```python
from build123d import *

# Parameters (mm, degrees)
ARMB_W_DEPTH             = 19.5
FILLET_1_R               = 16
FILLET_2_R               = 10
CUT_EXTRUDE_1_DEPTH      = 169.89419765
CUT_EXTRUDE_1_DEPTH_BACK = 169.89419765
SKETCH_2_R               = 10
CUT_EXTRUDE_2_DEPTH      = 169.89419765
CUT_EXTRUDE_2_DEPTH_BACK = 169.89419765
ARMB_T_W                 = 35
ARMB_T_H                 = 18
CUT_EXTRUDE_3_DEPTH      = 169.89419765
SKETCH_5_R               = 4
SKETCH_5_R_2             = 3.25
CUT_EXTRUDE_4_DEPTH      = 173.238207143
SKETCH_6_R               = 3
CUT_EXTRUDE_5_DEPTH      = 171.133036181
CHAMFER_1_SIZE           = 0.2


with BuildPart() as part:
    # ArmB-L → ArmB-W (new, symmetric)
    with BuildSketch(Plane.XY):
        with BuildLine():
            Line((12.489995997, 10), (167, 10))
            Line((167, 10), (167, -10))
            Line((167, -10), (12.489995997, -10))
            ThreePointArc((12.489995997, -10), (-16, 0), (12.489995997, 10))
        make_face()
    extrude(amount=ARMB_W_DEPTH, both=True)

    # ﾌｨﾚｯﾄ1
    fillet_1_edges = [part.edges().sort_by_distance(p)[0] for p in [
        (167, 10, 0),
    ]]
    fillet(fillet_1_edges, radius=FILLET_1_R)

    # ﾌｨﾚｯﾄ2
    fillet_2_edges = [part.edges().sort_by_distance(p)[0] for p in [
        (12.489995997, 10, 0),
        (12.489995997, -10, 0),
    ]]
    fillet(fillet_2_edges, radius=FILLET_2_R)

    # ｽｹｯﾁ2 → ｶｯﾄ - 押し出し1 (cut, two sides: drawn at the far end of the back side and taken through both)
    with BuildSketch(Plane.XY.offset(-CUT_EXTRUDE_1_DEPTH_BACK)):
        Circle(SKETCH_2_R)
    extrude(amount=CUT_EXTRUDE_1_DEPTH + CUT_EXTRUDE_1_DEPTH_BACK, mode=Mode.SUBTRACT)

    # ｽｹｯﾁ3 → ｶｯﾄ - 押し出し2 (cut, two sides: drawn at the far end of the back side and taken through both)
    with BuildSketch(Plane(origin=(0, 0, 0), x_dir=(1, 0, 0), z_dir=(0, 1, 0)).offset(-CUT_EXTRUDE_2_DEPTH_BACK)):
        with BuildLine():
            Line((-16, 17.5), (18.424067706, 17.5))
            ThreePointArc((18.424067706, 17.5), (26, 0), (18.424067706, -17.5))
            Line((18.424067706, -17.5), (-16, -17.5))
            Line((-16, -17.5), (-16, 17.5))
        make_face()
    extrude(amount=CUT_EXTRUDE_2_DEPTH + CUT_EXTRUDE_2_DEPTH_BACK, mode=Mode.SUBTRACT)

    # ArmB-t → ｶｯﾄ - 押し出し3 (cut, through all)
    with BuildSketch(Plane(origin=(0, 0, 0), x_dir=(0, 0, -1), z_dir=(1, 0, 0))):
        with Locations((0, 1)):
            Rectangle(ARMB_T_W, ARMB_T_H)
    extrude(amount=CUT_EXTRUDE_3_DEPTH, mode=Mode.SUBTRACT)

    # ｽｹｯﾁ5 → ｶｯﾄ - 押し出し4 (cut, through all)
    with BuildSketch(Plane.XY.offset(19.5)):
        with Locations((155, 3)):
            Circle(SKETCH_5_R)
        with Locations((139, 5)):
            Circle(SKETCH_5_R_2)
    extrude(amount=-CUT_EXTRUDE_4_DEPTH, mode=Mode.SUBTRACT)

    # ｽｹｯﾁ6 → ｶｯﾄ - 押し出し5 (cut, through all)
    with BuildSketch(Plane.XZ.offset(10)):
        with Locations(Location((155, 0, 0), (0, 0, 270))):
            Circle(SKETCH_6_R)
        with Locations(Location((40, 0, 0), (0, 0, 270))):
            Circle(SKETCH_6_R)
    extrude(amount=-CUT_EXTRUDE_5_DEPTH, mode=Mode.SUBTRACT)

    # 面取り1
    chamfer_1_edges = [part.edges().sort_by_distance(p)[0] for p in [
        (167, -8, 19.5),
        (151, 3, -19.5),
        (151, 3, -17.5),
        (151, 3, 17.5),
        (151, 3, 19.5),
        (135.75, 5, -19.5),
        (135.75, 5, -17.5),
        (135.75, 5, 17.5),
        (135.75, 5, 19.5),
        (155, -8, 3),
        (155, -10, 3),
        (40, -8, 3),
        (40, -10, 3),
        (83.806623863, 10, -19.5),
        (83.806623863, 10, 19.5),
        (162.313708499, 5.313708499, -19.5),
        (162.313708499, 5.313708499, 19.5),
        (91.806623863, -10, -19.5),
        (91.806623863, -10, 19.5),
        (-16, 0, -19.5),
        (-16, 0, 19.5),
        (13.216416623, -10.594600569, -19.5),
        (13.216416623, -10.594600569, 19.5),
        (13.216416623, 10.594600569, -19.5),
        (13.216416623, 10.594600569, 19.5),
        (-10, 0, -19.5),
        (-10, 0, 19.5),
        (167, -8, -19.5),
        (26, -10, 0),
        (-10, 0, -17.5),
        (17.518657716, -10, -17.5),
        (13.216416623, -10.594600569, -17.5),
        (-16, 0, -17.5),
        (13.216416623, 10.594600569, -17.5),
        (83.806623863, 10, -17.5),
        (-10, 0, 17.5),
        (13.216416623, -10.594600569, 17.5),
        (17.518657716, -10, 17.5),
        (83.806623863, 10, 17.5),
        (13.216416623, 10.594600569, 17.5),
        (-16, 0, 17.5),
        (167, -10, 0),
        (162.313708499, 5.313708499, 17.5),
        (162.313708499, 5.313708499, -17.5),
        (26, -8, 0),
        (167, -7, -17.5),
        (167, -7, 17.5),
        (167, -8, 0),
    ]]
    chamfer(chamfer_1_edges, length=CHAMFER_1_SIZE)


solid = part.part
```
Work out the finished part from the listing and answer in its coordinate system (mm). A direction names the side the tool comes from. Give positions to 0.01 mm unless a question says otherwise; leave off trailing zeros. Loops run counter-clockwise (first coordinate to the right, second up) from the corner with the lowest first, then second, coordinate; pieces in that order, holes last. Notation, with made-up numbers: (38, 14) -> (93, 14) arc R27 cw to (93, 40) -> close; hole circle Ø2 at (-11, -8). An arc over 180 degrees is marked (long way). Put each result on its own line as item: value. Start each with the question number.
Item 1: Each of these flat-tipped pins is pushed along its axis until it touches: P1, Ø6, axis at x = 102.5, z = -6, coming from the -Y side; P2, Ø0.5, axis at x = 83, z = 18.5, coming from the +Y side; P3, Ø5, axis at x = 40, z = 0, coming from the +Y side; P4, Ø10, axis at y = 5, z = 14, coming from the +X side. Where does it stop, or does it pass through?
Item 2: The mould has two halves that part along Z. Classify faces 3 (the face through (74, 0, 17.5)), 4 (the face through (158.815, 4.201, -18.489)): released by +Z, released by -Z, zero draft, split by the parting line, or undercut.
Item 3: The part is cut by section B-B (x = 139). State how many separate pieces and enclosed holes the cut face has, then the cut area to 3 significant figures.
Item 4: The part is cut by section C-C (x = 57). Give the vertices of the cut face in (y, z), then the cut area to 3 significant figures.
Item 5: Which of the six approach directions +Z, -Z, +X, -X, +Y, -Y give full straight-line access (tool end or side, diameter ignored) to faces 1 (the face through (92, -8, 0)), 2 (the face through (157.53, -9.01, -1.61))?
Item 6: The part is cut by section A-A (z = 0). Give the vertices of the cut face in (x, y), then the cut area to 3 significant figures.
Item 7: Find the intervals of material crossed by L1, parallel to X at y = -9.2, z = 0; L2, parallel to Z at x = 10, y = 9.5; L3, parallel to X at y = 0, z = 18.65, in increasing order. Write a range as [from, to].
Answers below:
1. P1: y = -10
1. P2: y = 10
1. P3: through
1. P4: x = 165.06
2. face 3: undercut
2. face 4: zero draft
3. separate pieces: 3
3. enclosed holes: 0
3. area: 124 mm2
4. outline: (-10, -19.3) -> (-9.8, -19.5) -> (9.8, -19.5) -> (10, -19.3) -> (10, -17.7) -> (9.8, -17.5) -> (-8, -17.5) -> (-8, 17.5) -> (9.8, 17.5) -> (10, 17.7) -> (10, 19.3) -> (9.8, 19.5) -> (-9.8, 19.5) -> (-10, 19.3) -> close
4. area: 150 mm2
5. face 1: +X, -X, +Y
5. face 2: +Y, -Y
6. outline: (26, -9.8) -> (26.2, -10) -> (36.8, -10) -> (37, -9.8) -> (37, -8.2) -> (36.8, -8) -> (26.2, -8) -> (26, -8.2) -> close; (43, -9.8) -> (43.2, -10) -> (151.8, -10) -> (152, -9.8) -> (152, -8.2) -> (151.8, -8) -> (43.2, -8) -> (43, -8.2) -> close; (158, -9.8) -> (158.2, -10) -> (166.8, -10) -> (167, -9.8) -> (167, -8.2) -> (166.8, -8) -> (158.2, -8) -> (158, -8.2) -> close
6. area: 258 mm2
7. L1: [26, 37], [43, 152], [158, 167]
7. L2: [-19.5, -17.5], [17.5, 19.5]
7. L3: [-16, -10], [10, 152.35], [157.65, 165.83]
